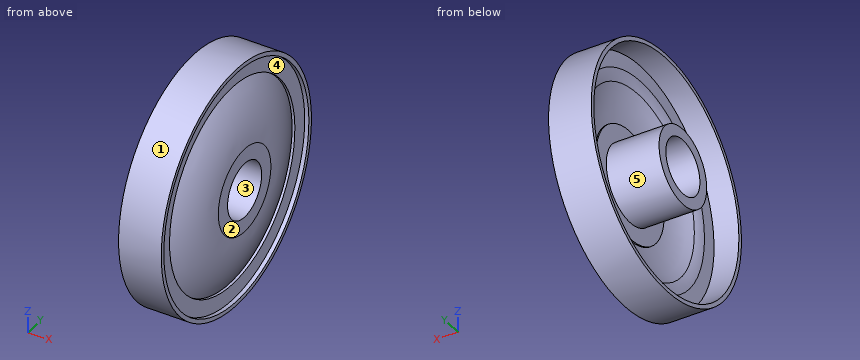
```python
from build123d import *

# Parameters (mm, degrees)
F2_R = 5


with BuildPart() as f1:
    # F0 (on Front) → F1 (revolve)
    with BuildSketch(Plane.XZ):
        with BuildLine():
            Line((3.865, 21.3), (3.865, 22.05))
            Line((3.865, 22.05), (-3.865, 22.05))
            Line((-3.865, 22.05), (-3.865, 21.3))
            Line((-3.865, 21.3), (0.634659, 21.3))
            Line((0.634659, 21.3), (0.634659, 17.269368))
            ThreePointArc((0.634659, 17.269368), (2.14433, 13.746856), (2.949481, 10))
            Line((2.949481, 10), (2.699481, 10))
            Line((2.699481, 10), (2.699481, 7))
            Line((2.699481, 7), (-6.865, 7))
            Line((-6.865, 7), (-6.865, 5))
            Line((-6.865, 5), (5.36081, 5))
            Line((5.36081, 5), (5.36081, 7.719591))
            ThreePointArc((5.36081, 7.719591), (4.663357, 13.233456), (2.614931, 18.399992))
            Line((2.614931, 18.399992), (3.115, 18.4))
            Line((3.115, 18.4), (3.115, 21.3))
            Line((3.115, 21.3), (3.865, 21.3))
        make_face()
    revolve(axis=Axis((-0.507669, 0, 0), (-1, 0, 0)))

    # F2
    f2_edges = [f1.edges().sort_by_distance(p)[0] for p in [
        (0.634659, 0, -17.269368),
    ]]
    fillet(f2_edges, radius=F2_R)


solid = f1.part
```
Model file for the job. Use its own axes, mm. Face numbers are marked on the shaded views. A direction names the side the tool comes from. Coordinates: 2 decimals unless noted, no trailing zeros. Order: outer loops, then holes, each group sorted by start corner. A loop starts at its lowest first (then second) coordinate and runs counter-clockwise, first axis right, second up. Notation, with made-up numbers: (-31, 89) -> (-11, 89) arc R16 cw to (-11, 107) -> close; hole circle Ø10 at (-8.5, 47.25). An arc over 180 degrees is marked (long way). Answer as a JSON object with one key per item and string values. Group by question number.
1) Pull direction Y, two halves, no side cores. Call the marked faces 1, 2 and 3: +Y half, -Y half, draft (parallel to the pull), parting line (faces both ways), or undercut.
2) Which spindle directions (+Z, -Z, +X, -X, +Y, -Y) get a long thin tool onto all of the face, cutting with end or side? Do the marked faces 4 and 5. Say none if no direction does.
3) Flat gauge pins, fed straight in: pin 1 (1.5 mm diameter, centred on x = 1, z = -2.5, fed in from -Y); pin 2 (6 mm diameter, centred on x = -1.5, z = -2.5, fed in from +Y); pin 3 (1.5 mm diameter, centred on x = -4.5, z = 12.5, fed in from +Y); pin 4 (1 mm diameter, centred on x = -5, y = 10, fed in from +Z). Where does each tip first touch, or does it go through?
4) Drill centre lines: L1, parallel to Y at x = -0.9, z = 0; L2, parallel to Y at x = 3.45, z = 0; L3, parallel to X at y = -8, z = -18 (3 decimals). Where is each one in solid material? Low to high.
5) Cut at A-A, the plane x = -2. Write the cut outline in (y, z), then the cut area to 3 significant figures.
Check values:
{
 "1": {"face 1": "parting line", "face 2": "draft", "face 3": "undercut"},
 "2": {"face 4": "+X", "face 5": "-X"},
 "3": {"pin 1": "stops at y = -21.98", "pin 2": "stops at y = 22.05", "pin 3": "stops at y = 18.43", "pin 4": "passes through"},
 "4": {"L1": "y = -22.05 to -21.3, -7 to -5, 5 to 7, 21.3 to 22.05", "L2": "y = -22.05 to -21.3, -16.72 to -5, 5 to 16.72, 21.3 to 22.05", "L3": "x = 0.635 to 3.115"},
 "5": {"outline": "circle Ø44.1 at (0, 0); circle Ø14 at (0, 0); hole circle Ø42.6 at (0, 0); hole circle Ø10 at (0, 0)", "area": "178 mm²"}
}
